from build123d import *

# Parameters (mm, degrees)
SKETCH1_W           = 12
SKETCH1_H           = 10.16
BOSS_EXTRUDE1_DEPTH = 8.64
FILLET1_R           = 1
SKETCH2_W           = 3.359416773
SKETCH2_H           = 0.86
BOSS_EXTRUDE2_DEPTH = 1


with BuildPart() as part:
    # Sketch1 → Boss-Extrude1 (new body)
    with BuildSketch(Plane.XY):
        with Locations((6, 5.08)):
            Rectangle(SKETCH1_W, SKETCH1_H)
    extrude(amount=BOSS_EXTRUDE1_DEPTH)

    # Fillet1
    fillet1_edges = [part.edges().sort_by_distance(p)[0] for p in [
        (12, 5.08, 8.64),
        (6, 10.16, 8.64),
        (0, 5.08, 8.64),
        (0, 10.16, 4.32),
        (12, 10.16, 4.32),
        (12, 0, 4.32),
        (0, 0, 4.32),
        (6, 0, 8.64),
    ]]
    fillet(fillet1_edges, radius=FILLET1_R)

    # Sketch2 → Boss-Extrude2 (add)
    with BuildSketch(Plane(origin=(0, 0, 0), x_dir=(-1, 0, 0), z_dir=(0, 0, -1))):
        with Locations((-11.000291613, 7.58)):
            Rectangle(SKETCH2_W, SKETCH2_H)
        with Locations((-11.000291613, 5.08)):
            Rectangle(SKETCH2_W, SKETCH2_H)
        with Locations((-11.000291613, 2.58)):
            Rectangle(SKETCH2_W, SKETCH2_H)
        with Locations((-0.999708387, 7.58)):
            Rectangle(SKETCH2_W, SKETCH2_H)
        with Locations((-0.999708387, 5.08)):
            Rectangle(SKETCH2_W, SKETCH2_H)
        with Locations((-0.999708387, 2.58)):
            Rectangle(SKETCH2_W, SKETCH2_H)
    extrude(amount=-BOSS_EXTRUDE2_DEPTH)


solid = part.part
Check sheet for the modelled part. Datum: model origin and axes. Units: mm. Give positions to 0.01 mm unless a question says otherwise; leave off trailing zeros. Order: outer loops, then holes, each group sorted by start corner. A loop starts at its lowest first (then second) coordinate and runs counter-clockwise, first axis right, second up. Notation, with made-up numbers: (9.25, 79) - (26.25, 79) arc R10 cw to (26.25, 93) - close; hole circle Ø1 at (-12.5, 15). An arc over 180 degrees is marked (long way). Answer as CSV lines item,"result".
1. Go/stop test with flat-tipped pins: P1, Ø0.5, axis at x = -0.5, z = 0.5, coming from the +Y side; P2, Ø2.5, axis at y = 6, z = 5, coming from the -X side; P3, Ø0.7, axis at x = 12.5, z = 0.5, coming from the -Y side. Record where each tip stops, or that it passes through.
Result sheet:
P1,"y = 8.01"
P2,"x = 0"
P3,"y = 2.15"
2. Section check D-D (y = 4.25). Record the boundary of the cut face in (x, z).
Result sheet:
outline,"(0, 0) - (12, 0) - (12, 7.64) arc R1 ccw to (11, 8.64) - (1, 8.64) arc R1 ccw to (0, 7.64) - close"
3. Scan lines: probe 1 along X at (y, z) = (6.5, 2.25); probe 2 along X at (y, z) = (5.5, 8.25); probe 3 along Z at (x, y) = (10.5, 0.75). Record each from-to range of solid material in increasing order. Write a range as from..to.
Result sheet:
probe 1,"0..12"
probe 2,"0.21..11.79"
probe 3,"0..8.61"
4. Section check A-A (y = 7.5). Record the boundary of the cut face in (x, z), then the cut area to 3 significant figures.
Result sheet:
outline,"(-0.68, 0) - (12.68, 0) - (12.68, 1) - (12, 1) - (12, 7.64) arc R1 ccw to (11, 8.64) - (1, 8.64) arc R1 ccw to (0, 7.64) - (0, 1) - (-0.68, 1) - close"
area,"105 mm²"
5. Section check C-C (x = 0.5). Record the boundary of the cut face in (y, z).
Result sheet:
outline,"(0.13, 0) - (10.03, 0) - (10.03, 7.64) arc R0.87 ccw to (9.16, 8.51) - (1, 8.51) arc R0.87 ccw to (0.13, 7.64) - close"
6. Section check B-B (z = 1.75). Record the boundary of the cut face in (x, y), then the cut area to 3 significant figures.
Result sheet:
outline,"(0, 1) arc R1 ccw to (1, 0) - (11, 0) arc R1 ccw to (12, 1) - (12, 9.16) arc R1 ccw to (11, 10.16) - (1, 10.16) arc R1 ccw to (0, 9.16) - close"
area,"121 mm²"
